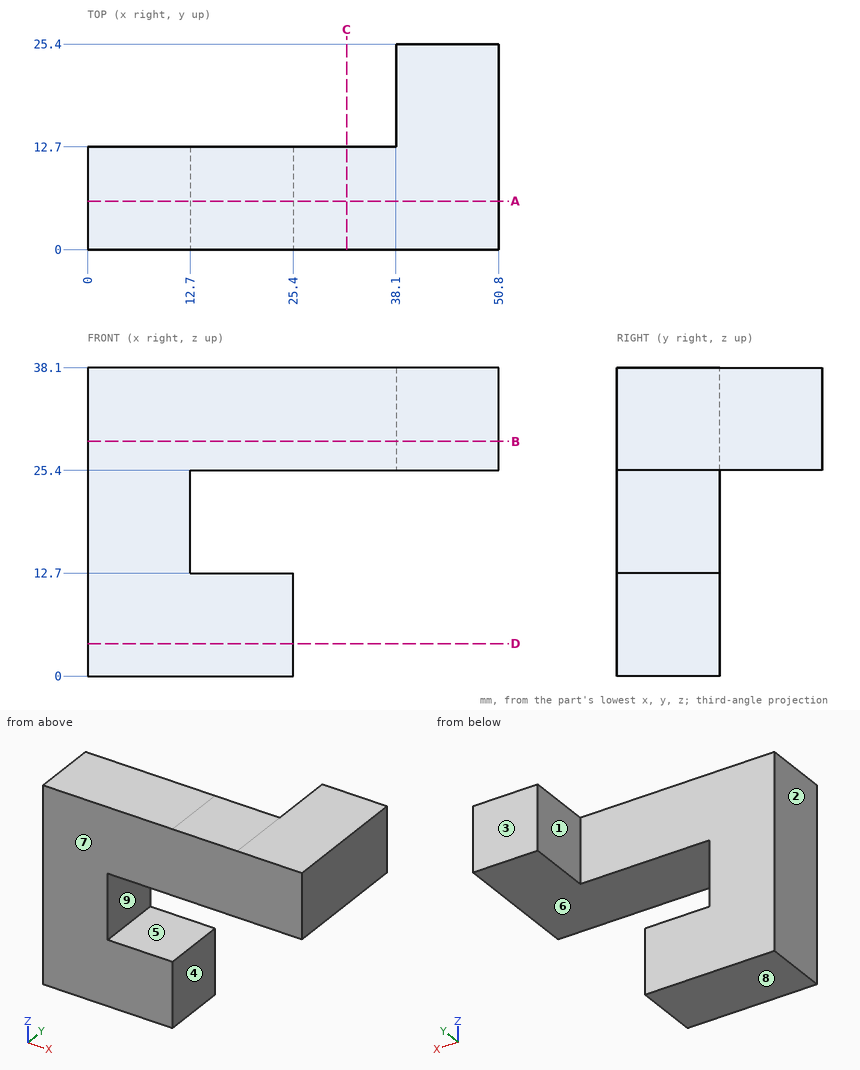
Verification items for this drawing (mm, ordinates from the low corner). A direction names the side the tool comes from. Give positions to 0.01 mm unless a question says otherwise; leave off trailing zeros. Loops run counter-clockwise (first coordinate to the right, second up) from the corner with the lowest first, then second, coordinate; pieces in that order, holes last. Notation, with made-up numbers: (40, 70.25) - (81, 70.25) arc R24 ccw to (81, 106.25) - close; hole circle Ø10 at (-2, -38.75). An arc over 180 degrees is marked (long way). Write item = value, one per line. Start each with the question number.
Q1. Mould release check, pull along Z, two halves, no side actions. Record for the marked faces 6, 7, 8 and 9: released by +Z, released by -Z, zero draft, split by the parting line, or undercut.
Q2. Depth check by flat-ended pin: P1, Ø6, axis at x = 41, y = 4.5, coming from the -Z side; P2, Ø1, axis at y = 14.5, z = 19, coming from the +X side; P3, Ø6, axis at y = 8.5, z = 13.5, coming from the +X side; P4, Ø4, axis at y = 18.5, z = 30, coming from the -X side. Enter the tip coordinate at first touch or a pass-through.
Q3. Cross-section at B-B, the plane z = 29. Enter the section's corners in (x, y), and give its area (3 significant figures).
Q4. Cross-section at D-D, the plane z = 4. Enter the section's corners in (x, y), and give its area (3 significant figures).
Q5. Thickness scan on line 1 (X direction, y = 11.5, z = 9); line 2 (X direction, y = 3.25, z = 15.5); line 3 (Z direction, x = 26, y = 10.25). Record the ranges inside material, lowest first.
Q6. Tool access check on the marked faces 1, 2, 3, 4 and 5. Record the directions out of +Z, -Z, +X, -X, +Y, -Y that give a thin tool (end or side, any length) a straight path to the whole face; none if there is none.
Q7. Cross-section at A-A, the plane y = 6. Enter the section's corners in (x, z), and give its area (3 significant figures).
Q8. Cross-section at C-C, the plane x = 32. Enter the section's corners in (y, z), and give its area (3 significant figures).
Answer key:
q1.face_6 = undercut
q1.face_7 = zero draft
q1.face_8 = released by -Z
q1.face_9 = undercut
q2.P1 = 25.4
q2.P2 = through
q2.P3 = 25.4
q2.P4 = 38.1
q3.outline = (0, 0) - (50.8, 0) - (50.8, 25.4) - (38.1, 25.4) - (38.1, 12.7) - (0, 12.7) - close
q3.area = 806 mm^2
q4.outline = (0, 0) - (25.4, 0) - (25.4, 12.7) - (0, 12.7) - close
q4.area = 323 mm^2
q5.line_1 = 0 to 25.4
q5.line_2 = 0 to 12.7
q5.line_3 = 25.4 to 38.1
q6.face_1 = +Z, -Z, -X, +Y
q6.face_2 = +Z, -Z, -X, +Y, -Y
q6.face_3 = +Z, -Z, +X, -X, +Y
q6.face_4 = -Z, +X, +Y, -Y
q6.face_5 = +X, +Y, -Y
q7.outline = (0, 0) - (25.4, 0) - (25.4, 12.7) - (12.7, 12.7) - (12.7, 25.4) - (50.8, 25.4) - (50.8, 38.1) - (38.1, 38.1) - (25.4, 38.1) - (0, 38.1) - close
q7.area = 1,130 mm^2
q8.outline = (0, 25.4) - (12.7, 25.4) - (12.7, 38.1) - (0, 38.1) - close
q8.area = 161 mm^2
